The model under review builds one solid part; all positions refer to its coordinate system, in mm. A direction names the side the tool comes from. Coordinates: 2 decimals unless noted, no trailing zeros. Write each loop counter-clockwise with the first axis right and the second up, starting at its lowest first coordinate (ties: lowest second). Pieces come first, ordered by that corner, then holes. Notation, with made-up numbers: (36.25, 41) - (69.25, 41) arc R23 ccw to (69.25, 65) - close; hole circle Ø3 at (24.5, 16). An arc over 180 degrees is marked (long way). Put each result on its own line as item: value.
from build123d import *

# Parameters (mm, degrees)
SKETCH1_W           = 23.3
SKETCH1_H           = 27.7
SKETCH1_W_2         = 17.3
SKETCH1_H_2         = 21.7
BOSS_EXTRUDE1_DEPTH = 13
SKETCH2_W           = 17.3
SKETCH2_H           = 21.7
SKETCH2_R           = 1.75
BOSS_EXTRUDE2_DEPTH = 2


with BuildPart() as part:
    # Sketch1 → Boss-Extrude1 (new body)
    with BuildSketch(Plane(origin=(0, 0, 0), x_dir=(1, 0, 0), z_dir=(0, 1, 0))):
        with Locations((0, 8.983417287)):
            Rectangle(SKETCH1_W, SKETCH1_H)
        with Locations((0, 8.983417287)):
            Rectangle(SKETCH1_W_2, SKETCH1_H_2, mode=Mode.SUBTRACT)
    extrude(amount=BOSS_EXTRUDE1_DEPTH)

    # Sketch2 → Boss-Extrude2 (add)
    with BuildSketch(Plane.XZ):
        with Locations((0, -8.983417287)):
            Rectangle(SKETCH2_W, SKETCH2_H)
        with Locations((6.24, -0.707949912)):
            Circle(SKETCH2_R, mode=Mode.SUBTRACT)
    extrude(amount=-BOSS_EXTRUDE2_DEPTH)


solid = part.part
1. The part is to be moulded in two halves that separate along Z. For faces 3 (the cylindrical face through (4.49, 0.99, -0.63)), 4 (the flat face through (0, 6, 4.867)), 5 (the flat face through (-11, 13, -9)), 6 (the flat face through (8.65, 7, -9)), say which applies: +Z half, -Z half, draft (parallel to the pull), parting line (faces both ways), or undercut.
Determined:
face 3: undercut
face 4: +Z half
face 5: draft
face 6: undercut
2. Machinability: for faces 1 (the flat face through (0, 6, -22.833)), 2 (the flat face through (0, 7, -19.833)), which of the approach directions +Z, -Z, +X, -X, +Y, -Y give a long, thin tool a straight path to every point of the face, cutting with its end or side? Answer none if there is none.
Determined:
face 1: -Z, +X, -X, +Y, -Y
face 2: +Y
3. To check wall thickness, follow probe 1 along X at (y, z) = (9, -2.5); probe 2 along Z at (x, y) = (7.75, 8.25); probe 3 along Z at (x, y) = (6.24, 0.9). State the ranges of each line that lie inside material, in increasing order.
Determined:
probe 1: x = -11.65 to -8.65, 8.65 to 11.65
probe 2: z = -22.83 to -19.83, 1.87 to 4.87
probe 3: z = -22.83 to -2.46, 1.04 to 4.87
4. Consider section A-A on y = 7. State the section outline as (x, z) points, plus the area to 3 significant figures.
Determined:
outline: (-11.65, -22.83) - (11.65, -22.83) - (11.65, 4.87) - (-11.65, 4.87) - close; hole (-8.65, -19.83) - (8.65, -19.83) - (8.65, 1.87) - (-8.65, 1.87) - close
area: 270 mm^2
5. Consider section C-C on x = -4. State the section outline as (y, z) points.
Determined:
outline: (0, -22.83) - (13, -22.83) - (13, -19.83) - (2, -19.83) - (2, 1.87) - (13, 1.87) - (13, 4.87) - (0, 4.87) - close
6. Consider section D-D on z = -16.5. State the section outline as (x, y) points, plus the area to 3 significant figures.
Determined:
outline: (-11.65, 0) - (11.65, 0) - (11.65, 13) - (8.65, 13) - (8.65, 2) - (-8.65, 2) - (-8.65, 13) - (-11.65, 13) - close
area: 113 mm^2
7. For pin 1 Ø12 at (x, z) = (2, -7.5) entering from +Y, flat-tipped, find the tip position at first contact; note if it passes through.
Determined:
pin 1: stops at y = 2
8. Consider section B-B on x = 6.24. State the section outline as (y, z) points.
Determined:
outline: (0, -22.83) - (13, -22.83) - (13, -19.83) - (2, -19.83) - (2, -2.46) - (0, -2.46) - close; (0, 1.04) - (2, 1.04) - (2, 1.87) - (13, 1.87) - (13, 4.87) - (0, 4.87) - close
